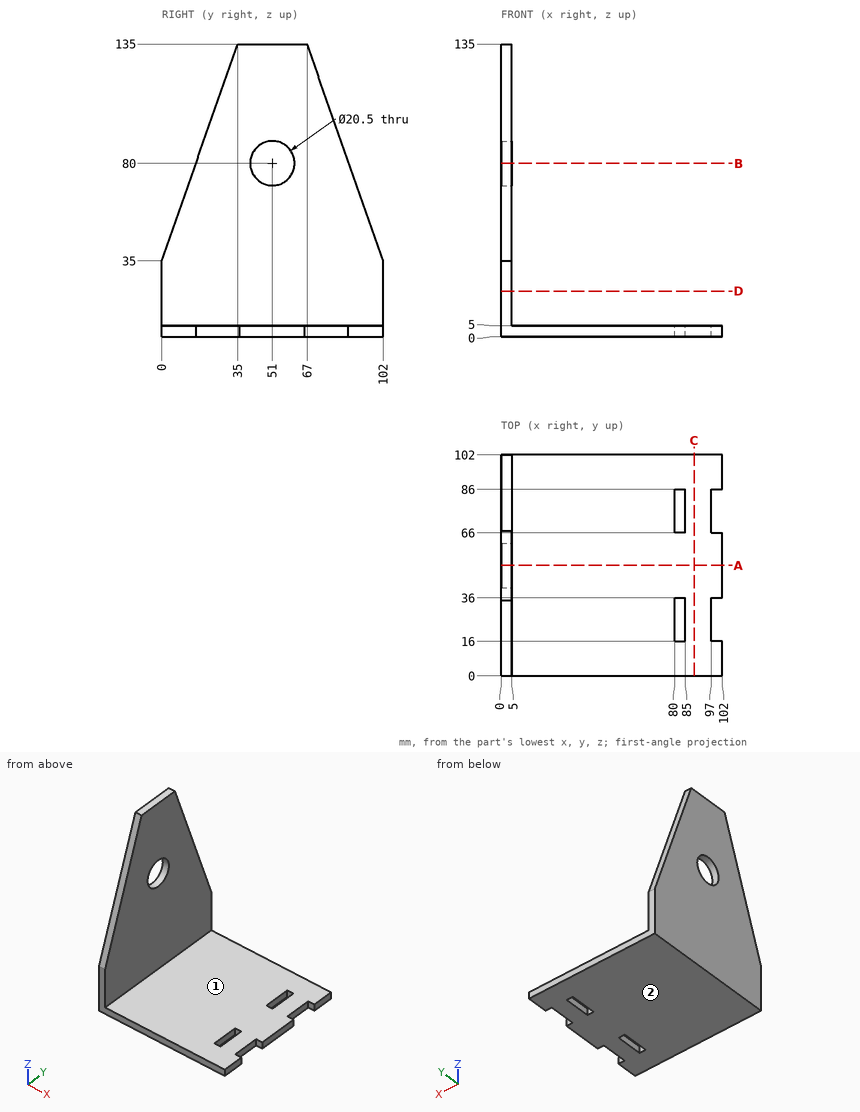
Study the drawing (mm; zero at the part's minimum x, y, z) and answer. A direction names the side the tool comes from. Coordinates: 2 decimals unless noted, no trailing zeros. Write each loop counter-clockwise with the first axis right and the second up, starting at its lowest first coordinate (ties: lowest second). Pieces come first, ordered by that corner, then holes. Notation, with made-up numbers: (-18, -30) - (15, -30) arc R26 ccw to (15, 0) - close; hole circle Ø2 at (24.25, -19). An arc over 180 degrees is marked (long way). Return JSON: item names as keys, results as strings. Group by question number.
1. Which of the six approach directions +Z, -Z, +X, -X, +Y, -Y give full straight-line access (tool end or side, diameter ignored) to the marked faces 1 and 2?
2. A cutting plane is placed at C-C, the plane x = 89. Determine the outline of the cut face in (y, z).
3. Straight lines are drawn through the part: L1, parallel to Z at x = 3.35, y = 51; L2, parallel to X at y = 23, z = 19.5. For each, find the intervals that lie inside material, in ascending order.
4. A cutting plane is placed at A-A, the plane y = 51. Determine the outline of the cut face in (x, z), plus the area to 3 significant figures.
5. A cutting plane is placed at D-D, the plane z = 21. Determine the outline of the cut face in (x, y), plus the area to 3 significant figures.
6. Given pin 1 (2 mm diameter, centred on y = 77.5, z = 27.5, fed in from +X); pin 2 (1.5 mm diameter, centred on y = 29.5, z = 2, fed in from +X); pin 3 (8 mm diameter, centred on x = 50.5, y = 33, fed in from +Z), each flat-ended and moving along its own axis, determine where each tip first touches the part or whether it passes through.
7. A cutting plane is placed at B-B, the plane z = 80. Determine the outline of the cut face in (x, y).
Ans:
{
 "1": {"face 1": "+Z, +X, +Y, -Y", "face 2": "-Z, +X, -X, +Y, -Y"},
 "2": {"outline": "(0, 0) - (102, 0) - (102, 5) - (0, 5) - close"},
 "3": {"L1": "0 to 69.75, 90.25 to 135", "L2": "0 to 5"},
 "4": {"outline": "(0, 0) - (102, 0) - (102, 5) - (5, 5) - (5, 69.75) - (0, 69.75) - close; (0, 90.25) - (5, 90.25) - (5, 135) - (0, 135) - close", "area": "1,060 mm²"},
 "5": {"outline": "(0, 0) - (5, 0) - (5, 102) - (0, 102) - close", "area": "510 mm²"},
 "6": {"pin 1": "x = 5", "pin 2": "x = 97", "pin 3": "z = 5"},
 "7": {"outline": "(0, 15.75) - (5, 15.75) - (5, 40.75) - (0, 40.75) - close; (0, 61.25) - (5, 61.25) - (5, 86.25) - (0, 86.25) - close"}
}
